```python
from build123d import *

# Parameters (mm, degrees)
BOSS_EXTRUDE1_DEPTH = 4


with BuildPart() as part:
    # Sketch1 → Boss-Extrude1 (new body)
    with BuildSketch(Plane(origin=(0, 0, 0), x_dir=(1, 0, 0), z_dir=(0, 1, 0))):
        Polygon((9.8625, 250), (-9.8625, 250), (-9.8625, 246), (-29.5875, 246), (-29.5875, 250), (-49.3125, 250), (-49.3125, 246), (-69.0375, 246), (-69.0375, 250), (-88.7625, 250), (-88.7625, 246), (-108.4875, 246), (-108.4875, 250), (-128.2125, 250), (-128.2125, 246), (-147.9375, 246), (-147.9375, 250), (-167.6625, 250), (-167.6625, 246), (-187.3875, 246), (-187.3875, 250), (-207.1125, 250), (-207.1125, 246), (-226.8375, 246), (-226.8375, 250), (-246.5625, 250), (-246.5625, 246), (-266.2875, 246), (-266.2875, 250), (-286.0125, 250), (-286.0125, 246), (-296.0125, 246), (-296.0125, 236), (-300.0125, 236), (-300.0125, 216.275), (-296.0125, 216.275), (-296.0125, 196.55), (-300.0125, 196.55), (-300.0125, 176.825), (-296.0125, 176.825), (-296.0125, 157.1), (-300.0125, 157.1), (-300.0125, 137.375), (-296.0125, 137.375), (-296.0125, 117.65), (-300.0125, 117.65), (-300.0125, 97.925), (-296.0125, 97.925), (-296.0125, 78.2), (-300.0125, 78.2), (-300.0125, 58.475), (-296.0125, 58.475), (-296.0125, 38.75), (-300.0125, 38.75), (-300.0125, 19.025), (-296.0125, 19.025), (-296.0125, 0), (296.0125, 0), (296.0125, 19.025), (300.0125, 19.025), (300.0125, 38.75), (296.0125, 38.75), (296.0125, 58.475), (300.0125, 58.475), (300.0125, 78.2), (296.0125, 78.2), (296.0125, 97.925), (300.0125, 97.925), (300.0125, 117.65), (296.0125, 117.65), (296.0125, 137.375), (300.0125, 137.375), (300.0125, 157.1), (296.0125, 157.1), (296.0125, 176.825), (300.0125, 176.825), (300.0125, 196.55), (296.0125, 196.55), (296.0125, 216.275), (300.0125, 216.275), (300.0125, 236), (296.0125, 236), (296.0125, 246), (286.0125, 246), (286.0125, 250), (266.2875, 250), (266.2875, 246), (246.5625, 246), (246.5625, 250), (226.8375, 250), (226.8375, 246), (207.1125, 246), (207.1125, 250), (187.3875, 250), (187.3875, 246), (167.6625, 246), (167.6625, 250), (147.9375, 250), (147.9375, 246), (128.2125, 246), (128.2125, 250), (108.4875, 250), (108.4875, 246), (88.7625, 246), (88.7625, 250), (69.0375, 250), (69.0375, 246), (49.3125, 246), (49.3125, 250), (29.5875, 250), (29.5875, 246), (9.8625, 246), align=None)
    extrude(amount=BOSS_EXTRUDE1_DEPTH)


solid = part.part
```
Input: part model. Units: mm. Frame: model coordinates. Coordinates: 2 decimals unless noted, no trailing zeros. Loops run counter-clockwise (first coordinate to the right, second up) from the corner with the lowest first, then second, coordinate; pieces in that order, holes last. Notation, with made-up numbers: M 70.25,30 L 81.25,30 A28 cw 81.25,52 Z; hole C 59.25,-5 d10. An arc over 180 degrees is marked long. One line per item, written item: value.
(1) Pin query (flat end, axial travel): pin 1 (2 mm diameter, centred on y = 1, z = -248, fed in from -X); pin 2 (2 mm diameter, centred on x = 288.5, y = 2.5, fed in from -Z); pin 3 (2 mm diameter, centred on x = 298, y = 2.5, fed in from -Z). Return the tip coordinate at first contact, or that it passes through.
Filled in:
pin 1: x = -286.01
pin 2: z = -246
pin 3: z = -236
(2) Line query: line 1 along X through (y, z) = (2.8, -87.5); line 2 along Z through (x, y) = (-226, 3). Output: solid intervals per line, ascending. Write a range as from..to.
Filled in:
line 1: -296.01..296.01
line 2: -246..0
(3) Section A-A (x = -213). Output: boundary loops of the cut face in (y, z).
Filled in:
outline: M 0,-246 L 4,-246 L 4,0 L 0,0 Z
